Could you check a few things on this drawing? It's one solid part, dimensions in mm from its lowest x, y, z. Give positions to 0.01 mm unless a question says otherwise; leave off trailing zeros. Loops run counter-clockwise (first coordinate to the right, second up) from the corner with the lowest first, then second, coordinate; pieces in that order, holes last. Notation, with made-up numbers: (57, 89.5) - (109, 89.5) arc R11 cw to (109, 100.5) - close; hole circle Ø7 at (-2, 82). An arc over 180 degrees is marked (long way). One line per item, written item: value. Start each with the question number.
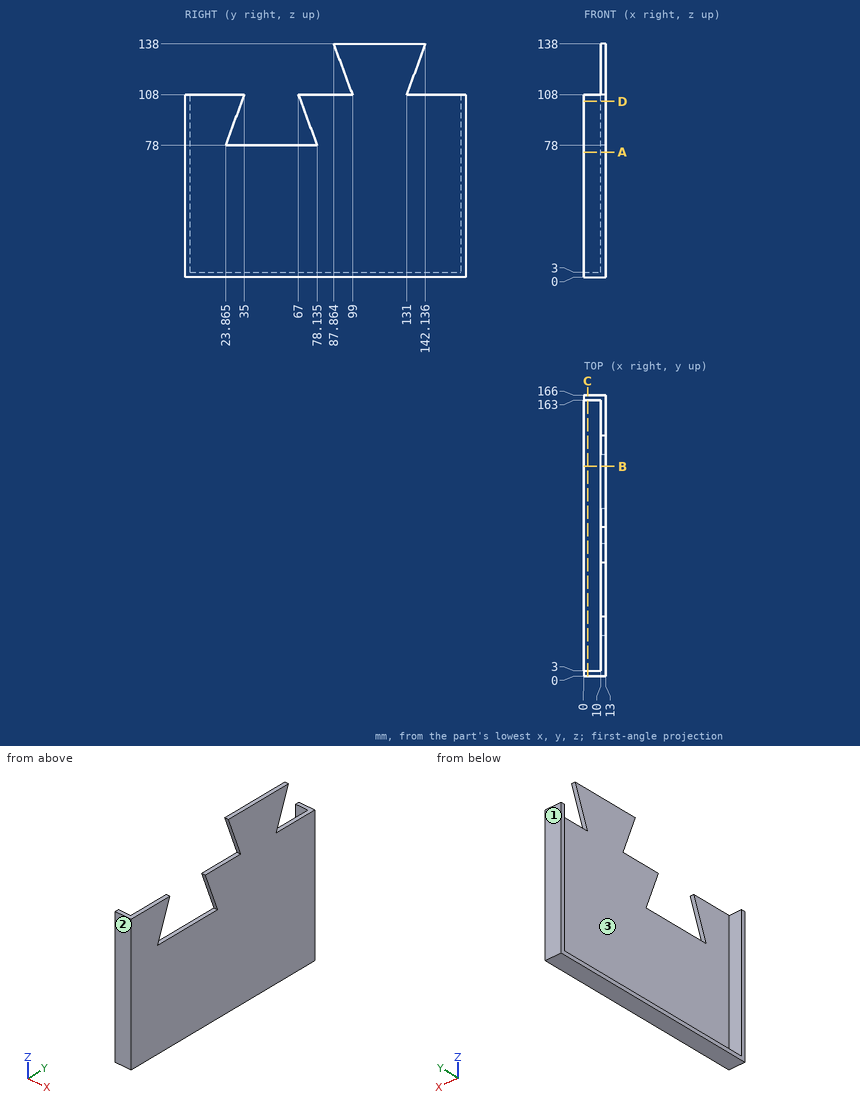
(1) If we section it at A-A on z = 74: List the corners of the cut face in (x, y) for me.
(2) If we mould it in two halves opening along Y, with no side actions, what happens to the marked faces 1, 2 and 3? For each: pulls with the +Y half, pulls with the -Y half, needs draft (parallel to the pull), parting line crosses it, or undercut.
(3) If we section it at D-D on z = 104: List the corners of the cut face in (x, y) for me (1 decimal).
(4) Will these pins go through, and if not, where does the flat tip stop? pin 1 (3.5 mm diameter, centred on x = 11, y = 45, fed in from +Z); pin 2 (5 mm diameter, centred on x = 6, y = 60.5, fed in from +Z); pin 3 (0.9 mm diameter, centred on x = 11, y = 82, fed in from +Z).
(5) If we section it at B-B on y = 124: List the corners of the cut face in (x, z) for me, plus the area to 3 significant figures.
(6) Please list where these lines run through material, in increasing order: probe 1 along Y at (x, z) = (8.25, 87); probe 2 along X at (y, z) = (104.5, 130.5); probe 3 along Z at (x, y) = (1.25, 89.5). Write a range as from..to.
(7) If we section it at C-C on x = 2.25: List the corners of the cut face in (y, z) for me, plus the area to 3 significant figures.
Found:
1. outline: (0, 0) - (13, 0) - (13, 166) - (0, 166) - (0, 163) - (10, 163) - (10, 3) - (0, 3) - close
2. face 1: pulls with the +Y half
2. face 2: pulls with the -Y half
2. face 3: undercut
3. outline: (0, 0) - (13, 0) - (13, 33.5) - (10, 33.5) - (10, 3) - (0, 3) - close; (0, 163) - (10, 163) - (10, 68.5) - (13, 68.5) - (13, 166) - (0, 166) - close
4. pin 1: z = 78
4. pin 2: z = 3
4. pin 3: z = 108
5. outline: (0, 0) - (13, 0) - (13, 138) - (10, 138) - (10, 3) - (0, 3) - close
5. area: 444 mm^2
6. probe 1: 0..3, 163..166
6. probe 2: 10..13
6. probe 3: 0..3
7. outline: (0, 0) - (166, 0) - (166, 108) - (163, 108) - (163, 3) - (3, 3) - (3, 108) - (0, 108) - close
7. area: 1,130 mm^2
